```python
from build123d import *

# Parameters (mm, degrees)
SKETCH2_W           = 558.8
SKETCH2_H           = 127
SKETCH2_R           = 5.08
BOSS_EXTRUDE1_DEPTH = 6.35
SKETCH3_R           = 2.1828125
CUT_EXTRUDE1_DEPTH  = 6.35


with BuildPart() as part:
    # Sketch2 → Boss-Extrude1 (new body)
    with BuildSketch(Plane(origin=(0, 0, 0), x_dir=(1, 0, 0), z_dir=(0, 1, 0))):
        with Locations((279.4, 63.5)):
            Rectangle(SKETCH2_W, SKETCH2_H)
        with Locations(Location((12.7, 63.5, 0), (0, 0, 270))):
            Circle(SKETCH2_R, mode=Mode.SUBTRACT)
        with Locations(Location((38.1, 63.5, 0), (0, 0, 270))):
            Circle(SKETCH2_R, mode=Mode.SUBTRACT)
        with Locations(Location((63.5, 63.5, 0), (0, 0, 270))):
            Circle(SKETCH2_R, mode=Mode.SUBTRACT)
        with Locations(Location((88.9, 63.5, 0), (0, 0, 270))):
            Circle(SKETCH2_R, mode=Mode.SUBTRACT)
        with Locations(Location((114.3, 63.5, 0), (0, 0, 270))):
            Circle(SKETCH2_R, mode=Mode.SUBTRACT)
        with Locations(Location((139.7, 63.5, 0), (0, 0, 270))):
            Circle(SKETCH2_R, mode=Mode.SUBTRACT)
        with Locations(Location((165.1, 63.5, 0), (0, 0, 270))):
            Circle(SKETCH2_R, mode=Mode.SUBTRACT)
        with Locations(Location((190.5, 63.5, 0), (0, 0, 270))):
            Circle(SKETCH2_R, mode=Mode.SUBTRACT)
        with Locations(Location((215.9, 63.5, 0), (0, 0, 270))):
            Circle(SKETCH2_R, mode=Mode.SUBTRACT)
        with Locations(Location((241.3, 63.5, 0), (0, 0, 270))):
            Circle(SKETCH2_R, mode=Mode.SUBTRACT)
        with Locations(Location((266.7, 63.5, 0), (0, 0, 270))):
            Circle(SKETCH2_R, mode=Mode.SUBTRACT)
        with Locations(Location((292.1, 63.5, 0), (0, 0, 270))):
            Circle(SKETCH2_R, mode=Mode.SUBTRACT)
        with Locations(Location((317.5, 63.5, 0), (0, 0, 270))):
            Circle(SKETCH2_R, mode=Mode.SUBTRACT)
        with Locations(Location((342.9, 63.5, 0), (0, 0, 270))):
            Circle(SKETCH2_R, mode=Mode.SUBTRACT)
        with Locations(Location((368.3, 63.5, 0), (0, 0, 270))):
            Circle(SKETCH2_R, mode=Mode.SUBTRACT)
        with Locations(Location((393.7, 63.5, 0), (0, 0, 270))):
            Circle(SKETCH2_R, mode=Mode.SUBTRACT)
        with Locations(Location((419.1, 63.5, 0), (0, 0, 270))):
            Circle(SKETCH2_R, mode=Mode.SUBTRACT)
        with Locations(Location((444.5, 63.5, 0), (0, 0, 270))):
            Circle(SKETCH2_R, mode=Mode.SUBTRACT)
        with Locations(Location((469.9, 63.5, 0), (0, 0, 270))):
            Circle(SKETCH2_R, mode=Mode.SUBTRACT)
        with Locations(Location((495.3, 63.5, 0), (0, 0, 270))):
            Circle(SKETCH2_R, mode=Mode.SUBTRACT)
        with Locations(Location((520.7, 63.5, 0), (0, 0, 270))):
            Circle(SKETCH2_R, mode=Mode.SUBTRACT)
        with Locations(Location((546.1, 63.5, 0), (0, 0, 270))):
            Circle(SKETCH2_R, mode=Mode.SUBTRACT)
    extrude(amount=BOSS_EXTRUDE1_DEPTH)

    # Sketch3 → Cut-Extrude1 (cut)
    with BuildSketch(Plane(origin=(0, 6.35, 0), x_dir=(1, 0, 0), z_dir=(0, 1, 0))):
        with Locations(Location((12.7, 120.65, 0), (0, 0, 270))):
            Circle(SKETCH3_R)
        with Locations(Location((139.7, 120.65, 0), (0, 0, 270))):
            Circle(SKETCH3_R)
        with Locations(Location((279.4, 120.65, 0), (0, 0, 270))):
            Circle(SKETCH3_R)
        with Locations(Location((419.1, 120.65, 0), (0, 0, 270))):
            Circle(SKETCH3_R)
        with Locations(Location((546.1, 120.65, 0), (0, 0, 270))):
            Circle(SKETCH3_R)
        with Locations(Location((546.1, 6.35, 0), (0, 0, 270))):
            Circle(SKETCH3_R)
        with Locations(Location((419.1, 6.35, 0), (0, 0, 270))):
            Circle(SKETCH3_R)
        with Locations(Location((279.4, 6.35, 0), (0, 0, 270))):
            Circle(SKETCH3_R)
        with Locations(Location((139.7, 6.35, 0), (0, 0, 270))):
            Circle(SKETCH3_R)
        with Locations(Location((12.7, 6.35, 0), (0, 0, 270))):
            Circle(SKETCH3_R)
    extrude(amount=-CUT_EXTRUDE1_DEPTH, mode=Mode.SUBTRACT)


solid = part.part
```
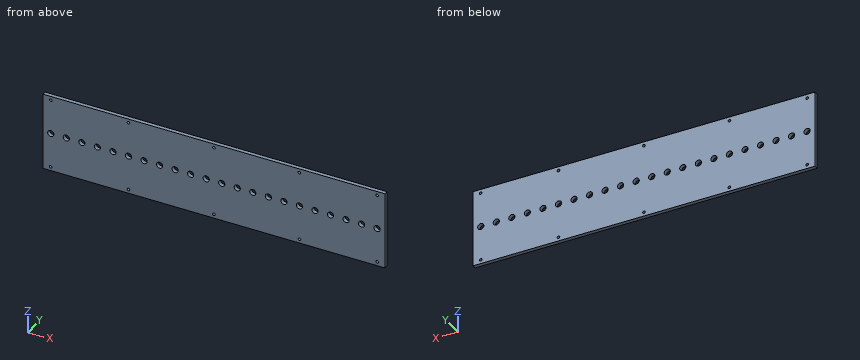
Could you check a few things on this model? Use its own coordinates, in mm. Give positions to 0.01 mm unless a question says otherwise; leave off trailing zeros. Write each loop counter-clockwise with the first axis right and the second up, starting at its lowest first coordinate (ties: lowest second). Pieces come first, ordered by that corner, then holes. Notation, with made-up numbers: (40, -22.5) - (75, -22.5) arc R17 cw to (75, 3.5) - close; hole circle Ø1 at (5, 34). An arc over 180 degrees is marked (long way). One line per item, written item: value. Start each with the question number.
Item 1: Please list where these lines run through material, in increasing order: line 1 (X direction, y = 4.75, z = -120.65); line 2 (Z direction, x = 393.7, y = 3.75); line 3 (Z direction, x = 446.5, y = 3.75). Write a range as from..to.
Item 2: I'm going to push a flat-ended pin straight in: pin 1 (6 mm diameter, centred on x = 165.1, z = -63.5, fed in from -Y) (1 decimal). Where does the tip first touch, or does it pass through?
Item 3: Imagine slicing it at B-B, the plane y = 3. Give the number of separate pieces and of enclosed holes in the cut face, and give its area (3 significant figures).
Item 4: Imagine slicing it at A-A, the plane x = 495.3. List the corners of the cut face in (y, z) for me.
Geometry says:
1. line 1: 0..10.52, 14.88..137.52, 141.88..277.22, 281.58..416.92, 421.28..543.92, 548.28..558.8
1. line 2: -127..-68.58, -58.42..0
1. line 3: -127..-68.17, -58.83..0
2. pin 1: through
3. separate pieces: 1
3. enclosed holes: 32
3. area: 69,000 mm^2
4. outline: (0, -127) - (6.35, -127) - (6.35, -68.58) - (0, -68.58) - close; (0, -58.42) - (6.35, -58.42) - (6.35, 0) - (0, 0) - close
